from build123d import *

# Parameters (mm, degrees)
SKETCH1_W           = 60
SKETCH1_H           = 10
BOSS_EXTRUDE1_DEPTH = 4
SKETCH2_R           = 1.75
CUT_EXTRUDE1_DEPTH  = 4
FILLET1_R           = 1


with BuildPart() as part:
    # Sketch1 → Boss-Extrude1 (new body)
    with BuildSketch(Plane(origin=(0, 0, 0), x_dir=(1, 0, 0), z_dir=(0, 1, 0))):
        Rectangle(SKETCH1_W, SKETCH1_H)
    extrude(amount=BOSS_EXTRUDE1_DEPTH)

    # Sketch2 → Cut-Extrude1 (cut)
    with BuildSketch(Plane(origin=(0, 4, 0), x_dir=(1, 0, 0), z_dir=(0, 1, 0))):
        with Locations(Location((-26, 0, 0), (0, 0, 270))):
            Circle(SKETCH2_R)
        with Locations(Location((7.5, 0, 0), (0, 0, 270))):
            Circle(SKETCH2_R)
        with Locations(Location((25, 0, 0), (0, 0, 270))):
            Circle(SKETCH2_R)
        with Locations(Location((-15, 0, 0), (0, 0, 270))):
            Circle(SKETCH2_R)
    extrude(amount=-CUT_EXTRUDE1_DEPTH, mode=Mode.SUBTRACT)

    # Fillet1
    fillet1_edges = [part.edges().sort_by_distance(p)[0] for p in [
        (-30, 4, 0),
        (0, 4, 5),
        (30, 4, 0),
        (0, 0, 5),
        (-30, 0, 0),
        (0, 0, -5),
        (30, 0, 0),
        (30, 2, 5),
        (-30, 2, 5),
        (-30, 2, -5),
        (30, 2, -5),
        (0, 4, -5),
    ]]
    fillet(fillet1_edges, radius=FILLET1_R)


solid = part.part
Input: part model. Units: mm. Frame: model coordinates. Coordinates: 2 decimals unless noted, no trailing zeros. Loops run counter-clockwise (first coordinate to the right, second up) from the corner with the lowest first, then second, coordinate; pieces in that order, holes last.
(1) Section D-D on x = -8.5. Return the cut outline in (y, z).
(2) Section A-A on z = 0. Return the cut outline in (x, y).
(3) Section C-C on y = 2.3. Return the cut outline in (x, z), then the cut area to 3 significant figures.
(4) Pull-direction query (Z, two-part tool) for faces 1 (the face through (30, 2, 0)), 2 (the face through (29.699, 2.014, 4.715)), 3 (the face through (26.735, 2.028, -0.228)); classes: released by +Z, released by -Z, zero draft, split by the parting line, or undercut.
(5) Material intervals for probe 1 along X at (y, z) = (1.7, 0); probe 2 along X at (y, z) = (1.7, -1.5); probe 3 along Z at (x, y) = (1, 0.95), sorted ascending.
(6) First-contact query: pin 1 Ø3 at (x, z) = (-15, 0) entering from +Y; pin 2 Ø5.5 at (x, z) = (7.5, 0) entering from +Y. Flat tips, straight axial feed; report the tip coordinate or a pass-through.
(7) Section B-B on x = -26. Return the cut outline in (y, z).
Data:
1. outline: (0, -4) arc R1 ccw to (1, -5) - (3, -5) arc R1 ccw to (4, -4) - (4, 4) arc R1 ccw to (3, 5) - (1, 5) arc R1 ccw to (0, 4) - close
2. outline: (-30, 1) arc R1 ccw to (-29, 0) - (-27.75, 0) - (-27.75, 4) - (-29, 4) arc R1 ccw to (-30, 3) - close; (-24.25, 0) - (-16.75, 0) - (-16.75, 4) - (-24.25, 4) - close; (-13.25, 0) - (5.75, 0) - (5.75, 4) - (-13.25, 4) - close; (9.25, 0) - (23.25, 0) - (23.25, 4) - (9.25, 4) - close; (26.75, 0) - (29, 0) arc R1 ccw to (30, 1) - (30, 3) arc R1 ccw to (29, 4) - (26.75, 4) - close
3. outline: (-30, -4) arc R1 ccw to (-29, -5) - (29, -5) arc R1 ccw to (30, -4) - (30, 4) arc R1 ccw to (29, 5) - (-29, 5) arc R1 ccw to (-30, 4) - close; hole circle Ø3.5 at (-26, 0); hole circle Ø3.5 at (-15, 0); hole circle Ø3.5 at (7.5, 0); hole circle Ø3.5 at (25, 0)
3. area: 561 mm2
4. face 1: zero draft
4. face 2: released by +Z
4. face 3: undercut
5. probe 1: x = -30 to -27.75, -24.25 to -16.75, -13.25 to 5.75, 9.25 to 23.25, 26.75 to 30
5. probe 2: x = -30 to -26.9, -25.1 to -15.9, -14.1 to 6.6, 8.4 to 24.1, 25.9 to 30
5. probe 3: z = -5 to 5
6. pin 1: passes through
6. pin 2: stops at y = 4
7. outline: (0, -4) arc R1 ccw to (1, -5) - (3, -5) arc R1 ccw to (4, -4) - (4, -1.75) - (0, -1.75) - close; (0, 1.75) - (4, 1.75) - (4, 4) arc R1 ccw to (3, 5) - (1, 5) arc R1 ccw to (0, 4) - close
